```python
from build123d import *

# Parameters (mm, degrees)
BOSS_EXTRUDE1_DEPTH = 10
BOSS_EXTRUDE2_DEPTH = 2.429285786
FILLET2_R           = 2


with BuildPart() as part:
    # Sketch2 → Boss-Extrude1 (new, symmetric)
    with BuildSketch(Plane.XY):
        Polygon((41.051421481, -27.990049876), (41.051421481, -48.990049876), (43.480707267, -48.990049876), (43.480707267, -61.778339755), (15.134736917, -64.258290817), (15.134736917, -69.258290817), (43.480707267, -71.738241879), (53.480707267, -71.738241879), (53.480707267, -27.990049876), align=None)
    extrude(amount=BOSS_EXTRUDE1_DEPTH, both=True)

    # Sketch4 → Boss-Extrude2 (add)
    with BuildSketch(Plane.ZY.offset(-43.480707267)):
        with BuildLine():
            Line((-10, -48.990049876), (-10, -58.990049876))
            ThreePointArc((-10, -58.990049876), (-7.071067812, -51.918982064), (0, -48.990049876))
            Line((0, -48.990049876), (-10, -48.990049876))
        make_face()
        with BuildLine():
            Line((10, -48.990049876), (0, -48.990049876))
            ThreePointArc((0, -48.990049876), (7.071067812, -51.918982064), (10, -58.990049876))
            Line((10, -58.990049876), (10, -48.990049876))
        make_face()
    extrude(amount=BOSS_EXTRUDE2_DEPTH)

    # Sketch3 → Cut-Revolve1 (revolve, cut)
    with BuildSketch(Plane.ZY.offset(-37.480707267)):
        with BuildLine():
            Line((-10, -44.490049876), (10, -44.490049876))
            Line((10, -44.490049876), (10, -29.490049876))
            ThreePointArc((10, -29.490049876), (0, -39.490049876), (-10, -29.490049876))
            Line((-10, -29.490049876), (-10, -44.490049876))
        make_face()
    revolve(axis=Axis((37.480707267, -44.490049876, -10), (0, 0, 1)), mode=Mode.SUBTRACT)

    # Fillet2
    fillet2_edges = [part.edges().sort_by_distance(p)[0] for p in [
        (53.480707267, -71.738241879, 0),
        (15.134736917, -69.258290817, 0),
        (15.134736917, -64.258290817, 0),
    ]]
    fillet(fillet2_edges, radius=FILLET2_R)


solid = part.part
```
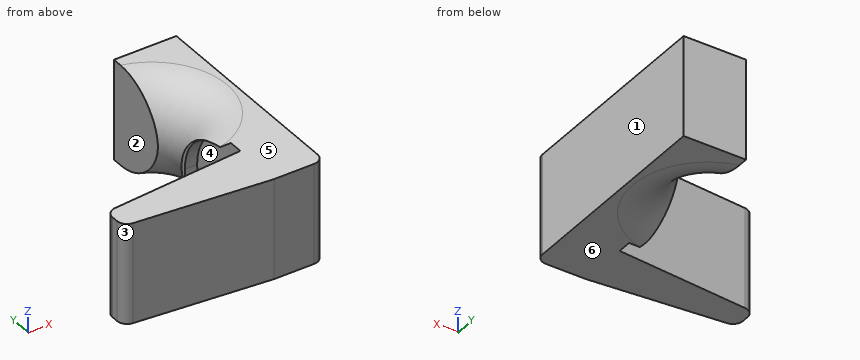
Part model, mm, in its own coordinate system. Face numbers are marked on the shaded views. A direction names the side the tool comes from. Round coordinates to 2 decimals unless told otherwise and drop trailing zeros. Order: outer loops, then holes, each group sorted by start corner. A loop starts at its lowest first (then second) coordinate and runs counter-clockwise, first axis right, second up. Notation, with made-up numbers: M 61,-7.75 L 72,-7.75 A18 cw 72,22.25 Z; hole C -24.5,-17.75 d1. An arc over 180 degrees is marked long. Put each result on its own line as item: value. Start each with the question number.
1. Tool access for the marked faces 1 and 2: list every direction of +Z, -Z, +X, -X, +Y, -Y with a clear straight run to the whole face (end or side of a thin tool).
2. Drop flat-ended pins along their axis: pin 1 (1.5 mm diameter, centred on y = -60.5, z = 2, fed in from -X); pin 2 (1 mm diameter, centred on y = -35.5, z = 3, fed in from -X); pin 3 (2 mm diameter, centred on x = 27, z = -4, fed in from +Y). Give the stop position or say it passes through.
3. Slice it at A-A on z = 6. List the corners of the cut face in (x, y), then the cut area to 3 significant figures.
4. Slice it at B-B on x = 22. List the corners of the cut face in (y, z).
5. Drill centre lines: probe 1 along X at (y, z) = (-61, 4); probe 2 along X at (y, z) = (-67.5, -3.75); probe 3 along Y at (x, z) = (43, -6.75). Where is each one in solid material? Low to high. Write a range as [from, to].
6. Two-plate mould, pull along Z, no slides. Class the marked faces 3, 4, 5 and 6: +Z half, -Z half, draft (parallel to the pull), parting line (faces both ways), or undercut.
7. Slice it at D-D on y = -63. List the corners of the cut face in (x, z).
8. Slice it at C-C on z = 8.5. List the corners of the cut face in (x, y).
Findings:
1. face 1: +Z, -Z, +X, +Y, -Y
1. face 2: +Z, -Z, -X, +Y
2. pin 1: x = 43.48
2. pin 2: x = 41.05
2. pin 3: y = -63.13
3. outline: M 15.13,-67.43 A2 ccw 16.96,-69.42 L 43.48,-71.74 L 51.48,-71.74 A2 ccw 53.48,-69.74 L 53.48,-27.99 L 41.05,-27.99 L 41.05,-38.47 A7 cw 41.05,-50.51 L 41.05,-50.99 L 43.48,-50.99 L 43.48,-61.78 L 16.96,-64.1 A2 ccw 15.13,-66.09 Z
3. area: 674 mm2
4. outline: M -69.86,-10 L -63.66,-10 L -63.66,10 L -69.86,10 Z
5. probe 1: [43.48, 53.48]
5. probe 2: [15.14, 53.48]
5. probe 3: [-71.7, -61.82], [-51.61, -49.75], [-39.23, -27.99]
6. face 3: draft
6. face 4: undercut
6. face 5: +Z half
6. face 6: -Z half
7. outline: M 29.52,-10 L 53.48,-10 L 53.48,10 L 29.52,10 Z
8. outline: M 15.13,-67.43 A2 ccw 16.96,-69.42 L 43.48,-71.74 L 51.48,-71.74 A2 ccw 53.48,-69.74 L 53.48,-27.99 L 41.05,-27.99 L 41.05,-35.44 A9.73 cw 41.05,-53.54 L 41.05,-53.72 L 43.48,-53.72 L 43.48,-61.78 L 16.96,-64.1 A2 ccw 15.13,-66.09 Z
